Build history of the part. All positions in model axes, mm. Face numbers are marked on the shaded views. A direction names the side the tool comes from. Give positions to 0.01 mm unless a question says otherwise; leave off trailing zeros. Write each loop counter-clockwise with the first axis right and the second up, starting at its lowest first coordinate (ties: lowest second). Pieces come first, ordered by that corner, then holes. Notation, with made-up numbers: (-20, 25) -> (20, 25) arc R10 cw to (20, 34) -> close; hole circle Ø4 at (4.5, -14). An arc over 180 degrees is marked (long way). Put each result on its own line as item: value. Start each with the question number.
Item 1: Flat gauge pins, fed straight in: pin 1 Ø2.5 at (y, z) = (5.27, -3.3) entering from +X; pin 2 Ø1 at (x, z) = (6, -1) entering from -Y; pin 3 Ø5.5 at (y, z) = (-9, -4) entering from -X. Where does each tip first touch, or does it go through?
Item 2: Tool access for the marked faces 5 and 6: list every direction of +Z, -Z, +X, -X, +Y, -Y with a clear straight run to the whole face (end or side of a thin tool).
Item 3: Two-plate mould, pull along Y, no slides. Class the marked faces 1, 2, 3 and 4: pulls with the +Y half, pulls with the -Y half, needs draft (parallel to the pull), parting line crosses it, or undercut.
Item 4: Drill centre lines: line 1 along Y through (x, z) = (7.5, -3.3); line 2 along Y through (x, z) = (2.5, -3.3); line 3 along X through (y, z) = (-9.5, -1.5). Where is each one in solid material? Low to high.
Item 5: Slice it at D-D, the plane y = -11. List the corners of the cut face in (x, z), plus the area to 3 significant figures.
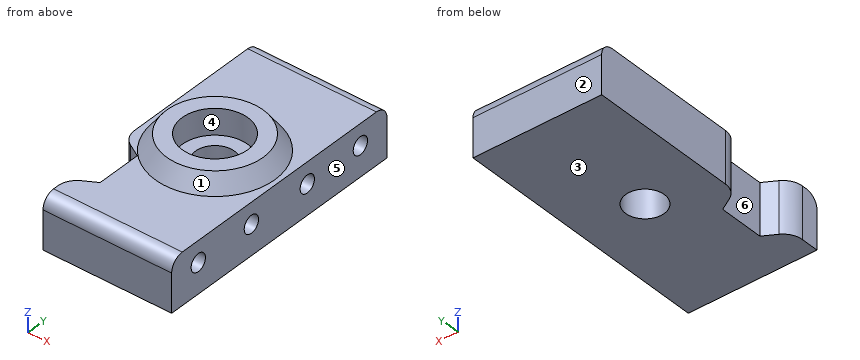
```python
from build123d import *
from OCP.BRepFilletAPI import BRepFilletAPI_MakeChamfer

# Parameters (mm, degrees)
SKETCH1_W           = 20
SKETCH1_H           = 40.56076
BOSS_EXTRUDE1_DEPTH = 8
SKETCH6_R           = 1.35
CUT_EXTRUDE1_DEPTH  = 10
SKETCH8_R           = 7.5
BOSS_EXTRUDE2_DEPTH = 2.5
SKETCH9_R           = 5.1
CUT_EXTRUDE3_DEPTH  = 4
SKETCH10_R          = 3
CUT_EXTRUDE4_DEPTH  = 6.5
FILLET1_R           = 2
CHAMFER1_SIZE2      = 2.5
CHAMFER1_SIZE       = 1.8
SKETCH11_W          = 8
SKETCH11_H          = 7
CUT_EXTRUDE5_DEPTH  = 3.5
CHAMFER2_SIZE       = 2.020725942
CHAMFER2_SIZE_2     = 3.5
FILLET2_R           = 3


with BuildPart() as part:
    # Sketch1 → Boss-Extrude1 (new body)
    with BuildSketch(Plane.XY):
        Rectangle(SKETCH1_W, SKETCH1_H)
    extrude(amount=-BOSS_EXTRUDE1_DEPTH)

    # Sketch6 → Cut-Extrude1 (cut)
    with BuildSketch(Plane(origin=(10, 0, 0), x_dir=(0, 0, -1), z_dir=(1, 0, 0))):
        with Locations(Location((3.3, -15.26519, 0), (0, 0, 180))):
            Circle(SKETCH6_R)
        with Locations((3.3, -5.26519)):
            Circle(SKETCH6_R)
        with Locations((3.3, 15.26519)):
            Circle(SKETCH6_R)
        with Locations(Location((3.3, 5.26519, 0), (0, 0, 180))):
            Circle(SKETCH6_R)
    extrude(amount=-CUT_EXTRUDE1_DEPTH, mode=Mode.SUBTRACT)

    # Sketch8 → Boss-Extrude2 (add)
    with BuildSketch(Plane.XY):
        Circle(SKETCH8_R)
    extrude(amount=BOSS_EXTRUDE2_DEPTH)

    # Sketch9 → Cut-Extrude3 (cut)
    with BuildSketch(Plane.XY.offset(2.5)):
        Circle(SKETCH9_R)
    extrude(amount=-CUT_EXTRUDE3_DEPTH, mode=Mode.SUBTRACT)

    # Sketch10 → Cut-Extrude4 (cut)
    with BuildSketch(Plane.XY.offset(-1.5)):
        Circle(SKETCH10_R)
    extrude(amount=-CUT_EXTRUDE4_DEPTH, mode=Mode.SUBTRACT)

    # Fillet1
    fillet1_edges = [part.edges().sort_by_distance(p)[0] for p in [
        (0, -20.28038, 0),
        (0, 20.28038, 0),
    ]]
    fillet(fillet1_edges, radius=FILLET1_R)

    # Chamfer1
    chamfer1_edges = [part.edges().sort_by_distance(p)[0] for p in [
        (-7.5, 0, 0),
    ]]
    chamfer1_side = [part.faces().sort_by_distance(p)[0] for p in [
        (-7.536, 0, 0),
    ]]
    chamfer(chamfer1_edges, length=CHAMFER1_SIZE - 0.0001, length2=CHAMFER1_SIZE2 - 0.0001, reference=chamfer1_side[0])  # a hair under: the kernel refuses the full size

    # Sketch11 → Cut-Extrude5 (cut)
    with BuildSketch(Plane.ZY.offset(10)):
        with Locations((-4, -10.26517)):
            Rectangle(SKETCH11_W, SKETCH11_H)
    extrude(amount=-CUT_EXTRUDE5_DEPTH, mode=Mode.SUBTRACT)

    # Chamfer2
    chamfer2_edges_1 = [part.edges().sort_by_distance(p)[0] for p in [
        (-10, -13.76517, -4),
    ]]
    chamfer2_side_1 = [part.faces().sort_by_distance(p)[0] for p in [
        (-10, -13.805584519, -4),
    ]]
    chamfer2_edges_2 = [part.edges().sort_by_distance(p)[0] for p in [
        (-10, -6.76517, -4),
    ]]
    chamfer2_side_2 = [part.faces().sort_by_distance(p)[0] for p in [
        (-9.959585481, -6.76517, -4),
    ]]
    chamfer2 = BRepFilletAPI_MakeChamfer(part.part.solid().wrapped)
    for e in chamfer2_edges_1:
        chamfer2.Add(CHAMFER2_SIZE - 0.0001, CHAMFER2_SIZE_2 - 0.0001, e.wrapped, chamfer2_side_1[0].wrapped)
    for e in chamfer2_edges_2:
        chamfer2.Add(CHAMFER2_SIZE_2 - 0.0001, CHAMFER2_SIZE - 0.0001, e.wrapped, chamfer2_side_2[0].wrapped)
    add(Compound.cast(chamfer2.Shape()), mode=Mode.REPLACE)  # a hair under: the kernel refuses the full size

    # Fillet2
    fillet2_edges = [part.edges().sort_by_distance(p)[0] for p in [
        (-10, -15.785795942, -4),
        (-10, -4.744544058, -4),
    ]]
    fillet(fillet2_edges, radius=FILLET2_R)


solid = part.part
```
Values follow:
1. pin 1: x = 0
1. pin 2: y = -20.22
1. pin 3: x = -7.39
2. face 5: +Z, -Z, +X, +Y, -Y
2. face 6: +Z, -Z, -X
3. face 1: parting line crosses it
3. face 2: pulls with the +Y half
3. face 3: needs draft
3. face 4: undercut
4. line 1: -20.28 to -16.62, -13.92 to -6.62, -3.92 to 3.92, 6.62 to 13.92, 16.62 to 20.28
4. line 2: -20.28 to -16.62, -13.92 to -6.62, -3.92 to -1.66, 1.66 to 3.92, 6.62 to 13.92, 16.62 to 20.28
4. line 3: -6.5 to 10
5. outline: (-6.5, -8) -> (10, -8) -> (10, 0) -> (-6.5, 0) -> close
5. area: 132 mm2
